```python
from build123d import *

# Parameters (mm, degrees)
SKETCH004_W   = 50
SKETCH004_H   = 25
SKETCH004_W_2 = 45.5
SKETCH004_H_2 = 21
PAD001_DEPTH  = 10
SKETCH003_R   = 0.9
PAD002_DEPTH  = 6
SKETCH005_W   = 50
SKETCH005_H   = 25
SKETCH005_R   = 8.5
PAD003_DEPTH  = 2
SKETCH006_W   = 12
SKETCH006_H   = 2
POCKET_DEPTH  = 2


with BuildPart() as part:
    # Sketch004 (on DatumPlane) → Pad001 (new body)
    with BuildSketch(Plane(origin=(-8.845912, -3.712389, 7.5), x_dir=(1, 0, 0), z_dir=(0, 1, 0))):
        Rectangle(SKETCH004_W, SKETCH004_H)
        Rectangle(SKETCH004_W_2, SKETCH004_H_2, mode=Mode.SUBTRACT)
    extrude(amount=PAD001_DEPTH)

    # Sketch003 (on DatumPlane) → Pad002 (join)
    with BuildSketch(Plane(origin=(-8.845912, -3.712389, 7.5), x_dir=(1, 0, 0), z_dir=(0, 1, 0))):
        with BuildLine():
            Line((-23.5, -10.75), (-14.5, -10.75))
            Line((-14.5, -8.3666), (-14.5, -10.75))
            ThreePointArc((-15.5, 8.124038), (-21.484415, -0.514499), (-14.5, -8.3666))
            Line((-15.5, 10.75), (-15.5, 8.124038))
            Line((-15.5, 10.75), (-23.5, 10.75))
            Line((-23.5, 10.75), (-23.5, -10.75))
        make_face()
        with Locations((-21, 8.7)):
            Circle(SKETCH003_R, mode=Mode.SUBTRACT)
        with Locations((-21, -8.7)):
            Circle(SKETCH003_R, mode=Mode.SUBTRACT)
        with BuildLine():
            Line((23.5, -10.75), (23.5, 10.75))
            Line((23.5, 10.75), (14.5, 10.75))
            Line((14.5, 8.3666), (14.5, 10.75))
            ThreePointArc((14.5, -8.3666), (21.5, 0), (14.5, 8.3666))
            Line((14.5, -8.3666), (14.5, -10.75))
            Line((14.5, -10.75), (23.5, -10.75))
        make_face()
        with Locations((21, -8.7)):
            Circle(SKETCH003_R, mode=Mode.SUBTRACT)
        with Locations((21, 8.7)):
            Circle(SKETCH003_R, mode=Mode.SUBTRACT)
    extrude(amount=PAD002_DEPTH)

    # Sketch005 (on DatumPlane) → Pad003 (join)
    with BuildSketch(Plane(origin=(-8.845912, -3.712389, 7.5), x_dir=(1, 0, 0), z_dir=(0, 1, 0))):
        Rectangle(SKETCH005_W, SKETCH005_H)
        with Locations((-13, 0)):
            Circle(SKETCH005_R, mode=Mode.SUBTRACT)
        with Locations((13, 0)):
            Circle(SKETCH005_R, mode=Mode.SUBTRACT)
    extrude(amount=PAD003_DEPTH)

    # Sketch006 (on Face11 of Pad003) → Pocket (cut)
    with BuildSketch(Plane(origin=(-8.845912, 6.287611, 7.5), x_dir=(1, 0, 0), z_dir=(0, 1, 0))):
        with Locations((0, 11.5)):
            Rectangle(SKETCH006_W, SKETCH006_H)
    extrude(amount=-POCKET_DEPTH, mode=Mode.SUBTRACT)


with BuildPart() as part_1:
    # Body001 placement: moved
    add(part.part.moved(Location((24, 0, 0))))


solid = part_1.part
```
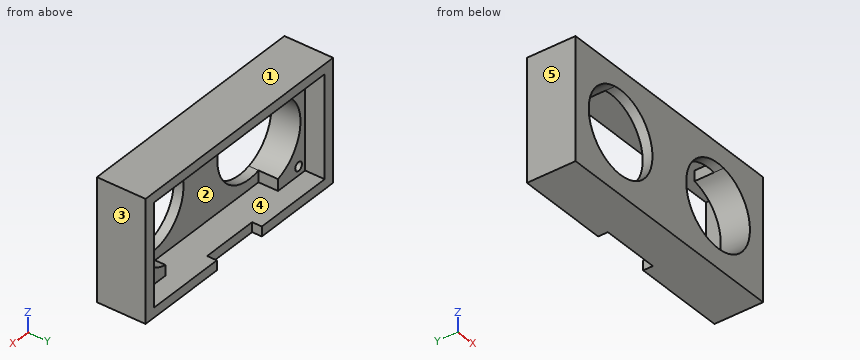
Geometry check sheet. Reference: the model listing, model coordinates, mm. Face numbers are marked on the shaded views. A direction names the side the tool comes from. Coordinates: 2 decimals unless noted, no trailing zeros. Order: outer loops, then holes, each group sorted by start corner. A loop starts at its lowest first (then second) coordinate and runs counter-clockwise, first axis right, second up. Notation, with made-up numbers: M 28,1 L 87,1 A19 ccw 87,19 Z; hole C 70.5,66 d7. An arc over 180 degrees is marked long. One line per question, with ' | ' between items. Start each with the question number.
Item 1: Cross-section at D-D on x = 28. Enter the section's corners in (y, z), then the cut area to 3 significant figures.
Item 2: Gauge pin test, flat ends, axial feed: pin 1 (2.5 mm diameter, centred on x = -5.85, z = 16.2, fed in from +Y); pin 2 (4 mm diameter, centred on x = 32, z = 10.5, fed in from +Y); pin 3 (1.6 mm diameter, centred on x = 15.5, z = -4, fed in from +Y); pin 4 (5 mm diameter, centred on x = 9.5, z = 0, fed in from +Y). Record the tip position at first contact, or that the pin passes through.
Item 3: Cross-section at A-A on y = 3.75. Enter the section's corners in (x, z), then the cut area to 4 significant figures.
Item 4: Set-up check for the marked faces 4 and 5: record each of +Z, -Z, +X, -X, +Y, -Y from which the full face is reachable in a straight line by a thin tool's end or side.
Item 5: Material ranges on L1, parallel to X at y = 0.8, z = 16.2; L2, parallel to X at y = -2.95, z = 7.5; L3, parallel to X at y = 3.5, z = -2.75, recorded low to high. Write a range as [from, to].
Item 6: Draft check along X on the marked faces 1, 2 and 3. Enter one of: pulls with the +X half, pulls with the -X half, needs draft (parallel to the pull), parting line crosses it, or undercut.
Item 7: Cross-section at C-C on y = -1. Enter the section's corners in (x, z).
Item 8: Cross-section at B-B on z = 7.5. Enter the section's corners in (x, y).
Findings:
1) outline: M -3.71,-5 L 6.29,-5 L 6.29,-3 L -1.71,-3 L -1.71,-1 L -3.71,-1 Z; M -3.71,16 L -1.71,16 L -1.71,18 L 6.29,18 L 6.29,20 L -3.71,20 Z | area: 48.0 mm²
2) pin 1: stops at y = 2.29 | pin 2: passes through | pin 3: stops at y = 4.29 | pin 4: stops at y = -1.71
3) outline: M -9.85,-5 L 40.15,-5 L 40.15,20 L -9.85,20 Z; hole M -7.6,-3 L 37.9,-3 L 37.9,18 L -7.6,18 Z | area: 294.5 mm²
4) face 4: +Y | face 5: +Z, -Z, -X, +Y, -Y
5) L1: x = [-9.85, -6.75], [-4.95, 0.65], [29.65, 35.25], [37.05, 40.15] | L2: x = [-9.85, -6.35], [10.65, 19.65], [36.65, 40.15] | L3: x = [-9.85, -7.6], [37.9, 40.15]
6) face 1: needs draft | face 2: undercut | face 3: pulls with the +X half
7) outline: M -9.85,-5 L 40.15,-5 L 40.15,20 L -9.85,20 Z; hole C -5.85,-1.2 d1.8; hole C -5.85,16.2 d1.8; hole M -0.35,-3 L 29.65,-3 L 29.65,-0.87 A8.5 ccw 29.65,15.87 L 29.65,18 L 0.65,18 L 0.65,15.87 A8.5 ccw -0.35,-0.62 Z; hole C 36.15,-1.2 d1.8; hole C 36.15,16.2 d1.8
8) outline: M -9.85,-3.71 L -6.35,-3.71 L -6.35,2.29 L -7.6,2.29 L -7.6,6.29 L -9.85,6.29 Z; M 10.65,-3.71 L 19.65,-3.71 L 19.65,-1.71 L 10.65,-1.71 Z; M 36.65,-3.71 L 40.15,-3.71 L 40.15,6.29 L 37.9,6.29 L 37.9,2.29 L 36.65,2.29 Z
